```python
from build123d import *

# Parameters (mm, degrees)
F0_R          = 20
F1_DEPTH      = 5
F2_R          = 0.6
F3_DEPTH      = 5
F4_R          = 2.5
F5_DEPTH      = 15
F6_R          = 1
F7_DEPTH      = 25
F7_DEPTH_BACK = 25
F9_DEPTH      = 25
F9_DEPTH_BACK = 25
F8_R          = 5
F10_DEPTH     = 1
F11_R         = 10
F12_DEPTH     = 2.5


# Not quite as in the source:
# - a feature names something its author has since deleted; it is built from what else it names


with BuildPart() as f1:
    # F0 (on Front) → F1 (new body)
    with BuildSketch(Plane.XZ):
        Circle(F0_R)
    extrude(amount=F1_DEPTH)

    # F2 (on face) → F3 (cut, through all)
    with BuildSketch(Plane.XZ.offset(5)):
        with Locations((-13.23387, 0)):
            Circle(F2_R)
        with Locations((13.23387, 0)):
            Circle(F2_R)
    extrude(amount=-F3_DEPTH, mode=Mode.SUBTRACT)

    # F4 (on face) → F5 (join)
    with BuildSketch(Plane.XZ):
        Circle(F4_R)
    extrude(amount=-F5_DEPTH)

    # F6 (on Top) → F7 (cut, two sides)
    with BuildSketch(Plane.XY) as f7_sk:
        with Locations((0, 6.5963385438)):
            Circle(F6_R)
    extrude(amount=F7_DEPTH, mode=Mode.SUBTRACT)
    extrude(f7_sk.sketch, amount=-F7_DEPTH_BACK, mode=Mode.SUBTRACT)

    # F6 (on Top) → F9 (cut, two sides)
    with BuildSketch(Plane.XY) as f9_sk:
        with Locations((0, 6.5963385438)):
            Circle(F6_R)
    extrude(amount=-F9_DEPTH, mode=Mode.SUBTRACT)
    extrude(f9_sk.sketch, amount=F9_DEPTH_BACK, mode=Mode.SUBTRACT)

    # F8 (on face) → F10 (cut)
    with BuildSketch(Plane.XZ.offset(5)):
        Circle(F8_R)
    extrude(amount=-F10_DEPTH, mode=Mode.SUBTRACT)

    # F11 (on face) → F12 (join)
    with BuildSketch(Plane(origin=(0, 15, 0), x_dir=(-1, 0, 0), z_dir=(0, 1, 0))):
        Circle(F11_R)
    extrude(amount=-F12_DEPTH)


solid = f1.part
```
Part model, mm, in its own coordinate system. A direction names the side the tool comes from. Give positions to 0.01 mm unless a question says otherwise; leave off trailing zeros. Order: outer loops, then holes, each group sorted by start corner. A loop starts at its lowest first (then second) coordinate and runs counter-clockwise, first axis right, second up. Notation, with made-up numbers: M 5,39.5 L 18,39.5 A29 cw 18,73.5 Z; hole C 10,74 d3. An arc over 180 degrees is marked long. Use a Markdown table: item, result. Add a question column.
(1) Saw through at A-A, the plane x = 0. Give the cut face in (y, z), and give its area (4 significant figures).
(2) Saw through at B-B, the plane z = -4.5. Give the cut face in (x, y).
(3) 3-axis set-ups, long thin cutter, end or side, ignore diameter. For faces 5 (the face through (-13.833, -2.535, 0.026)), 6 (the face through (0, -4, 0)), 7 (the face through (-2, 12.5, -2)), 8 (the face through (0, 15, 0)), 9 (the face through (2.17, 13.77, -9.76)): which of +Z, -Z, +X, -X, +Y, -Y reach the whole face in a straight line?
(4) Drop flat-ended pins along their axis: P1, Ø3, axis at x = 0, y = 6.6, coming from the -Z side; P2, Ø1.5, axis at x = 8, y = -2.5, coming from the +Z side; P3, Ø8, axis at x = 0, y = 5.5, coming from the +Z side; P4, Ø1.6, axis at x = -13.23, z = 0, coming from the -Y side. Give the stop position or say it passes through.
(5) Saw through at D-D, the plane x = -4. Give the cut face in (y, z).
(6) Probe line 1 along Y through (x, z) = (0, -1); line 2 along Z through (x, y) = (0, -4.5); line 3 along Y through (x, z) = (-2, 6.5). List the from-to ranges inside material, lowest first. Write a range as [from, to].
(7) Mould opens along Z. For faces 1 (the face through (4, -5, -4)), 2 (the face through (12.76, -2.54, -0.37)), 3 (the face through (2.385, 6.162, 0.751)), 4 (the face through (-1.08, -4.51, -4.88)) say: +Z half, -Z half, draft (parallel to the pull), parting line (faces both ways), or undercut.
(8) Saw through at C-C, the plane y = 11.5. Give the cut face in (x, z).
Answer key:
| question | item | result |
|---|---|---|
| 1 | outline | M -5,-20 L 0,-20 L 0,-2.5 L 5.6,-2.5 L 5.6,2.5 L 0,2.5 L 0,20 L -5,20 L -5,5 L -4,5 L -4,-5 L -5,-5 Z; M 7.6,-2.5 L 12.5,-2.5 L 12.5,-10 L 15,-10 L 15,10 L 12.5,10 L 12.5,2.5 L 7.6,2.5 Z |
| 1 | area | 292.5 mm^2 |
| 2 | outline | M -19.49,-5 L -2.18,-5 L -2.18,-4 L 2.18,-4 L 2.18,-5 L 19.49,-5 L 19.49,0 L -19.49,0 Z; M -8.93,12.5 L 8.93,12.5 L 8.93,15 L -8.93,15 Z |
| 3 | face 5 | +Y, -Y |
| 3 | face 6 | -Y |
| 3 | face 7 | none |
| 3 | face 8 | +Z, -Z, +X, -X, +Y |
| 3 | face 9 | +Y |
| 4 | P1 | z = -2.5 |
| 4 | P2 | z = 18.64 |
| 4 | P3 | z = 2.5 |
| 4 | P4 | y = -5 |
| 5 | outline | M -5,-19.6 L 0,-19.6 L 0,19.6 L -5,19.6 L -5,3 L -4,3 L -4,-3 L -5,-3 Z; M 12.5,-9.17 L 15,-9.17 L 15,9.17 L 12.5,9.17 Z |
| 6 | line 1 | [-4, 5.6], [7.6, 15] |
| 6 | line 2 | [-20, -5], [5, 20] |
| 6 | line 3 | [-5, 0], [12.5, 15] |
| 7 | face 1 | draft |
| 7 | face 2 | undercut |
| 7 | face 3 | parting line |
| 7 | face 4 | undercut |
| 8 | outline | C 0,0 d5 |
